Verification items for the finished model (mm, model axes). A direction names the side the tool comes from. Coordinates: 2 decimals unless noted, no trailing zeros. Write each loop counter-clockwise with the first axis right and the second up, starting at its lowest first coordinate (ties: lowest second). Pieces come first, ordered by that corner, then holes.
```python
from build123d import *

# Parameters (mm, degrees)
SKETCH_1_R          = 25
EXTRUDE_1_DEPTH     = 8
SKETCH_7_R          = 14.05
CUT_EXTRUDE_6_DEPTH = 6
SKETCH_2_R          = 4.5
CUT_EXTRUDE_7_DEPTH = 11.5


with BuildPart() as part:
    # 草圖1 → 填料-伸長1 (new body)
    with BuildSketch(Plane.XY):
        Circle(SKETCH_1_R)
    extrude(amount=EXTRUDE_1_DEPTH)

    # 草圖7 → 除料-伸長6 (cut)
    with BuildSketch(Plane.XY.offset(8)):
        Circle(SKETCH_7_R)
    extrude(amount=-CUT_EXTRUDE_6_DEPTH, mode=Mode.SUBTRACT)

    # 草圖2 → 除料-伸長7 (cut)
    with BuildSketch(Plane.XY):
        Circle(SKETCH_2_R)
    extrude(amount=CUT_EXTRUDE_7_DEPTH, mode=Mode.SUBTRACT)


solid = part.part
```
1. Material ranges on L1, parallel to Y at x = 0, z = 6.3; L2, parallel to Y at x = 0, z = 1.5; L3, parallel to X at y = 11, z = 5.75, recorded low to high.
2. Draft check along X on faces 1 (the cylindrical face through (-0.59, 4.46, 0.99)), 2 (the flat face through (11, -11, 8)), 3 (the cylindrical face through (23.846, 7.509, 3.944)). Enter one of: pulls with the +X half, pulls with the -X half, needs draft (parallel to the pull), parting line crosses it, or undercut.
3. Sectioned sample at D-D, the plane y = 11. Record the boundary of the cut face in (x, z).
4. Tool access check on faces 4 (the cylindrical face through (-3.046, -13.716, 5.042)), 5 (the flat face through (0, -5, 0)). Record the directions out of +Z, -Z, +X, -X, +Y, -Y that give a thin tool (end or side, any length) a straight path to the whole face; none if there is none.
5. Gauge pin test, flat ends, axial feed: P1, Ø22.5, axis at x = 2.5, y = 1, coming from the +Z side; P2, Ø3, axis at y = -10.5, z = 6.5, coming from the +X side; P3, Ø2, axis at x = 19.5, z = 4, coming from the +Y side; P4, Ø5.5, axis at x = 0, y = 0, coming from the +Z side. Record the tip position at first contact, or that the pin passes through.
6. Sectioned sample at A-A, the plane x = 0. Record the boundary of the cut face in (y, z), and give its area (3 significant figures).
7. Sectioned sample at C-C, the plane z = 6.25. Record the boundary of the cut face in (x, y), and give its area (3 significant figures).
Outcome:
1. L1: y = -25 to -14.05, 14.05 to 25
1. L2: y = -25 to -4.5, 4.5 to 25
1. L3: x = -22.45 to -8.74, 8.74 to 22.45
2. face 1: undercut
2. face 2: needs draft
2. face 3: parting line crosses it
3. outline: (-22.45, 0) - (22.45, 0) - (22.45, 8) - (8.74, 8) - (8.74, 2) - (-8.74, 2) - (-8.74, 8) - (-22.45, 8) - close
4. face 4: +Z
4. face 5: -Z, +X, -X, +Y, -Y
5. P1: stops at z = 2
5. P2: stops at x = 23.32
5. P3: stops at y = 16.82
5. P4: passes through
6. outline: (-25, 0) - (-4.5, 0) - (-4.5, 2) - (-14.05, 2) - (-14.05, 8) - (-25, 8) - close; (4.5, 0) - (25, 0) - (25, 8) - (14.05, 8) - (14.05, 2) - (4.5, 2) - close
6. area: 213 mm2
7. outline: circle Ø50 at (0, 0); hole circle Ø28.1 at (0, 0)
7. area: 1,340 mm2
